Geometry: final body of the model. Coordinates: model frame, mm. Face numbers are marked on the shaded views. A direction names the side the tool comes from. Coordinates: 2 decimals unless noted, no trailing zeros. Write each loop counter-clockwise with the first axis right and the second up, starting at its lowest first coordinate (ties: lowest second). Pieces come first, ordered by that corner, then holes. Notation, with made-up numbers: (65, 37) - (101, 37) arc R29 ccw to (101, 59) - close; hole circle Ø11 at (50.25, 33.5). An arc over 180 degrees is marked (long way). Put each result on its own line as item: value.
```python
from build123d import *

# Parameters (mm, degrees)
F0_W     = 101.6
F0_H     = 63.5
F1_DEPTH = 25.4
F2_R     = 6.35
F3_DEPTH = 25.401
F4_W     = 19.05
F4_H     = 38.1
F6_W     = 2.54
F6_H     = 12.7


with BuildPart() as f1:
    # F0 (on Top) → F1 (new body)
    with BuildSketch(Plane.XY):
        Rectangle(F0_W, F0_H)
    extrude(amount=F1_DEPTH)

    # F2 (on face) → F3 (cut, through all)
    with BuildSketch(Plane.XY.offset(25.4)):
        with Locations((-38.1, 19.05)):
            Circle(F2_R)
        with Locations((-38.1, -19.05)):
            Circle(F2_R)
        with Locations((38.1, 19.05)):
            Circle(F2_R)
        with Locations((38.1, -19.05)):
            Circle(F2_R)
    extrude(amount=-F3_DEPTH, mode=Mode.SUBTRACT)

    # F4 (on Front) → F5 (revolve)
    with BuildSketch(Plane.XZ):
        with Locations((-9.525, 44.45)):
            Rectangle(F4_W, F4_H)
    revolve(axis=Axis((0, 0, 44.45), (0, 0, -1)))

    # F6 (on Front) → F8 (revolve, cut)
    with BuildSketch(Plane.XZ):
        with Locations((-17.78, 44.45)):
            Rectangle(F6_W, F6_H)
    revolve(axis=Axis((0, 0, 44.295382), (0, 0, -1)), mode=Mode.SUBTRACT)


solid = f1.part
```
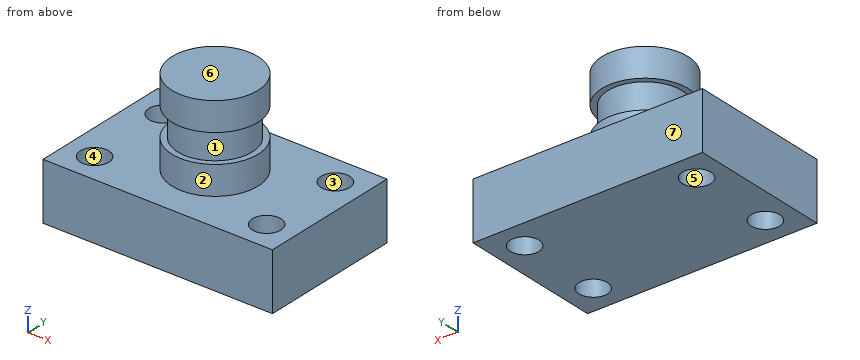
1. Section query C-C (y = -15). Return loops of the section in (x, z), then the cut area to 3 significant figures.
Answer below:
outline: (-50.8, 0) - (-42.99, 0) - (-42.99, 25.4) - (-50.8, 25.4) - close; (-33.21, 0) - (33.21, 0) - (33.21, 25.4) - (11.74, 25.4) - (11.74, 38.1) - (6.9, 38.1) - (6.9, 50.8) - (11.74, 50.8) - (11.74, 63.5) - (-11.74, 63.5) - (-11.74, 50.8) - (-6.9, 50.8) - (-6.9, 38.1) - (-11.74, 38.1) - (-11.74, 25.4) - (-33.21, 25.4) - close; (42.99, 0) - (50.8, 0) - (50.8, 25.4) - (42.99, 25.4) - close
area: 2,860 mm²
2. Pin query (flat end, axial travel): pin 1 Ø4 at (y, z) = (-9, 48) entering from +X; pin 2 Ø16.5 at (x, y) = (38.1, -19.05) entering from +Z; pin 3 Ø1 at (y, z) = (11.5, 43) entering from +X. Return the tip coordinate at first contact, or that it passes through.
Answer below:
pin 1: stops at x = 14.95
pin 2: stops at z = 25.4
pin 3: stops at x = 12.31
3. Section query B-B (z = 12). Return loops of the section in (x, y), then the cut area to 3 significant figures.
Answer below:
outline: (-50.8, -31.75) - (50.8, -31.75) - (50.8, 31.75) - (-50.8, 31.75) - close; hole circle Ø12.7 at (-38.1, -19.05); hole circle Ø12.7 at (-38.1, 19.05); hole circle Ø12.7 at (38.1, -19.05); hole circle Ø12.7 at (38.1, 19.05)
area: 5,940 mm²
4. Mould query, pull axis Y, two halves, no side actions, for the marked faces 4, 5, 6 and 7. Classes: +Y half, -Y half, draft (parallel to the pull), parting line (faces both ways), or undercut.
Answer below:
face 4: undercut
face 5: undercut
face 6: draft
face 7: +Y half
5. Ray query, probe 1 along Y at (x, z) = (38.1, 11.75); probe 2 along X at (y, z) = (19.5, 16); probe 3 along Y at (x, z) = (-33, 20). Return the intervals inside material, ascending. Write a range as from..to.
Answer below:
probe 1: y = -31.75..-25.4, -12.7..12.7, 25.4..31.75
probe 2: x = -50.8..-44.43, -31.77..31.77, 44.43..50.8
probe 3: y = -31.75..-22.83, -15.27..15.27, 22.83..31.75
6. Section query D-D (y = 0). Return loops of the section in (x, z), then the cut area to 3 significant figures.
Answer below:
outline: (-50.8, 0) - (50.8, 0) - (50.8, 25.4) - (19.05, 25.4) - (19.05, 38.1) - (16.51, 38.1) - (16.51, 50.8) - (19.05, 50.8) - (19.05, 63.5) - (-19.05, 63.5) - (-19.05, 50.8) - (-16.51, 50.8) - (-16.51, 38.1) - (-19.05, 38.1) - (-19.05, 25.4) - (-50.8, 25.4) - close
area: 3,970 mm²
7. Set-up query: the marked faces 1, 2 and 3. Return all of +Z, -Z, +X, -X, +Y, -Y with unobstructed straight access to the full face (end or side cutting, diameter ignored); none if empty.
Answer below:
face 1: none
face 2: +Z
face 3: +Z, -Z
8. Section query A-A (x = -38.1). Return loops of the section in (y, z).
Answer below:
outline: (-31.75, 0) - (-25.4, 0) - (-25.4, 25.4) - (-31.75, 25.4) - close; (-12.7, 0) - (12.7, 0) - (12.7, 25.4) - (-12.7, 25.4) - close; (25.4, 0) - (31.75, 0) - (31.75, 25.4) - (25.4, 25.4) - close
